from build123d import *

# Parameters (mm, degrees)
F0_R     = 1.5875
F1_DEPTH = 4.7625
F3_DEPTH = 58.1406
F5_DEPTH = 69.215
F7_DEPTH = 25.4
F9_DEPTH = 4.7625


with BuildPart() as f1:
    # F0 (on Top) → F1 (new body)
    with BuildSketch(Plane.XY):
        Polygon((-17.145, 87.89836), (-42.545, 87.89836), (-42.545, 0), (-45.72, 0), (-45.72, -58.15164), (-42.545, -58.15164), (-42.545, -66.08914), (-34.6075, -66.08914), (-34.6075, -69.26414), (34.6075, -69.26414), (34.6075, -66.08914), (42.545, -66.08914), (42.545, -58.15164), (45.72, -58.15164), (45.72, 0), (42.545, 0), (42.545, 87.89836), (17.145, 87.89836), (17.145, 27.487862), (12.7, 27.487862), (12.7, 91.07336), (-12.7, 91.07336), (-12.7, 27.487862), (-17.145, 27.487862), align=None)
        with Locations((-31.75, -43.86414)):
            Circle(F0_R, mode=Mode.SUBTRACT)
        with Locations((31.75, -43.86414)):
            Circle(F0_R, mode=Mode.SUBTRACT)
        with Locations((-31.75, 57.73586)):
            Circle(F0_R, mode=Mode.SUBTRACT)
        with Locations((31.75, 57.73586)):
            Circle(F0_R, mode=Mode.SUBTRACT)
    extrude(amount=F1_DEPTH)

    # F2 (on face) → F3 (join)
    with BuildSketch(Plane.XZ.offset(58.15164)):
        with BuildLine():
            Line((-45.72, 20.0025), (-45.72, 4.7625))
            Line((-45.72, 4.7625), (-42.545, 4.7625))
            Line((-42.545, 4.7625), (-42.545, 20.0025))
            ThreePointArc((-42.545, 20.0025), (-42.225108, 20.927946), (-41.402, 21.458299))
            ThreePointArc((-41.402, 21.458299), (-40.126284, 23.045799), (-41.402, 24.633299))
            ThreePointArc((-41.402, 24.633299), (-44.485221, 23.179692), (-45.72, 20.0025))
        make_face()
        with BuildLine():
            Line((42.545, 20.0025), (42.545, 4.7625))
            Line((42.545, 4.7625), (45.72, 4.7625))
            Line((45.72, 4.7625), (45.72, 20.0025))
            ThreePointArc((45.72, 20.0025), (44.485221, 23.179692), (41.402, 24.633299))
            ThreePointArc((41.402, 24.633299), (40.126284, 23.045799), (41.402, 21.458299))
            ThreePointArc((41.402, 21.458299), (42.225108, 20.927946), (42.545, 20.0025))
        make_face()
    extrude(amount=-F3_DEPTH)

    # F4 (on face) → F5 (join)
    with BuildSketch(Plane.YZ.offset(34.6075)):
        with BuildLine():
            Line((-69.26414, 20.0025), (-69.26414, 4.7625))
            Line((-69.26414, 4.7625), (-66.08914, 4.7625))
            Line((-66.08914, 4.7625), (-66.08914, 20.0025))
            ThreePointArc((-66.08914, 20.0025), (-65.769247, 20.927946), (-64.94614, 21.458299))
            ThreePointArc((-64.94614, 21.458299), (-63.670424, 23.045799), (-64.94614, 24.633299))
            ThreePointArc((-64.94614, 24.633299), (-68.029361, 23.179692), (-69.26414, 20.0025))
        make_face()
    extrude(amount=-F5_DEPTH)

    # F6 (on face) → F7 (join)
    with BuildSketch(Plane.YZ.offset(12.7)):
        with BuildLine():
            Line((87.89836, 4.7625), (91.07336, 4.7625))
            Line((91.07336, 4.7625), (91.07336, 9.5377))
            ThreePointArc((91.07336, 9.5377), (89.48586, 11.1252), (87.89836, 9.5377))
            Line((87.89836, 9.5377), (87.89836, 4.7625))
        make_face()
    extrude(amount=-F7_DEPTH)

    # F8 (on face) → F9 (cut)
    with BuildSketch(Plane.XY.offset(4.7625)):
        Polygon((-33.281147, 83.13586), (-37.7825, 83.13586), (-37.7825, 78.634507), align=None)
        Polygon((-21.9075, 81.039123), (-21.9075, 83.13586), (-26.545955, 83.13586), (-37.7825, 71.899315), (-37.7825, 65.164123), align=None)
        Polygon((-12.869341, 22.725362), (-19.604533, 22.725362), (-37.7825, 4.547394), (-37.7825, -2.187798), align=None)
        Polygon((34.070774, 83.13586), (27.335582, 83.13586), (21.9075, 77.707778), (21.9075, 70.972586), align=None)
        Polygon((37.7825, 73.377202), (37.7825, 80.112394), (21.9075, 64.237394), (21.9075, 57.502202), align=None)
        Polygon((31.047308, -61.32664), (37.7825, -61.32664), (37.7825, -54.591448), align=None)
        with BuildLine():
            Line((-37.7825, -49.334142), (-37.7825, -56.069335))
            Line((-37.7825, -56.069335), (37.7825, 19.495665))
            Line((37.7825, 19.495665), (37.7825, 26.230858))
            Line((37.7825, 26.230858), (-29.803871, -41.355513))
            ThreePointArc((-29.803871, -41.355513), (-29.504936, -46.109204), (-34.258626, -45.810269))
            Line((-34.258626, -45.810269), (-37.7825, -49.334142))
        make_face()
        with BuildLine():
            ThreePointArc((32.535156, 54.659474), (29.918155, 55.142606), (28.588111, 57.447621))
            Line((28.588111, 57.447621), (21.9075, 50.76701))
            Line((21.9075, 50.76701), (21.9075, 44.031818))
            Line((21.9075, 44.031818), (32.535156, 54.659474))
        make_face()
        with BuildLine():
            ThreePointArc((-33.990248, 55.485991), (-33.995064, 59.980924), (-29.50013, 59.976109))
            Line((-29.50013, 59.976109), (-21.9075, 67.568739))
            Line((-21.9075, 67.568739), (-21.9075, 74.303931))
            Line((-21.9075, 74.303931), (-37.7825, 58.428931))
            Line((-37.7825, 58.428931), (-37.7825, 51.693739))
            Line((-37.7825, 51.693739), (-33.990248, 55.485991))
        make_face()
        with BuildLine():
            Line((17.576924, -61.32664), (24.312116, -61.32664))
            Line((24.312116, -61.32664), (37.7825, -47.856255))
            Line((37.7825, -47.856255), (37.7825, -41.121063))
            Line((37.7825, -41.121063), (34.92286, -43.980704))
            ThreePointArc((34.92286, -43.980704), (33.995064, -46.109204), (31.866564, -47.036999))
            Line((31.866564, -47.036999), (17.576924, -61.32664))
        make_face()
        with BuildLine():
            Line((4.10654, -61.32664), (10.841732, -61.32664))
            Line((10.841732, -61.32664), (28.587678, -43.580694))
            ThreePointArc((28.587678, -43.580694), (29.504936, -41.619076), (31.466554, -40.701817))
            Line((31.466554, -40.701817), (37.7825, -34.385871))
            Line((37.7825, -34.385871), (37.7825, -27.650679))
            Line((37.7825, -27.650679), (4.10654, -61.32664))
        make_face()
        Polygon((-9.363845, -61.32664), (-2.628653, -61.32664), (37.7825, -20.915487), (37.7825, -14.180295), align=None)
        Polygon((-22.834229, -61.32664), (-16.099037, -61.32664), (37.7825, -7.445103), (37.7825, -0.709911), align=None)
        Polygon((-36.304613, -61.32664), (-29.569421, -61.32664), (37.7825, 6.025281), (37.7825, 12.760473), align=None)
        Polygon((-37.7825, -35.863758), (-37.7825, -42.59895), (37.7825, 32.96605), (37.7825, 39.701242), (20.80662, 22.725362), align=None)
        Polygon((-37.7825, -22.393374), (-37.7825, -29.128566), (14.071428, 22.725362), (7.336236, 22.725362), align=None)
        Polygon((-37.7825, -8.92299), (-37.7825, -15.658182), (0.601044, 22.725362), (-6.134148, 22.725362), align=None)
        Polygon((-37.7825, 18.017778), (-37.7825, 11.282586), (-21.9075, 27.157586), (-21.9075, 33.892778), align=None)
        Polygon((-37.7825, 31.488163), (-37.7825, 24.752971), (-21.9075, 40.627971), (-21.9075, 47.363163), align=None)
        Polygon((-37.7825, 44.958547), (-37.7825, 38.223355), (-21.9075, 54.098355), (-21.9075, 60.833547), align=None)
        Polygon((37.7825, 46.436434), (37.7825, 53.171626), (21.9075, 37.296626), (21.9075, 30.561434), align=None)
        with BuildLine():
            Line((37.7825, 59.906818), (37.7825, 66.64201))
            Line((37.7825, 66.64201), (32.038239, 60.89775))
            ThreePointArc((32.038239, 60.89775), (34.343254, 59.567706), (34.826387, 56.950705))
            Line((34.826387, 56.950705), (37.7825, 59.906818))
        make_face()
    extrude(amount=-F9_DEPTH, mode=Mode.SUBTRACT)


solid = f1.part
The model under review builds one solid part; all positions refer to its coordinate system, in mm. A direction names the side the tool comes from. Give positions to 0.01 mm unless a question says otherwise; leave off trailing zeros. Loops run counter-clockwise (first coordinate to the right, second up) from the corner with the lowest first, then second, coordinate; pieces in that order, holes last. Notation, with made-up numbers: (-20.5, -24) -> (8.5, -24) arc R12 ccw to (8.5, -9) -> close; hole circle Ø3 at (-15, 37.25). An arc over 180 degrees is marked (long way). Answer as a JSON object with one key per item and string values. Group by question number.
Q1. Draft analysis for pull direction X (two halves, no side actions). For faces 4 (the flat face through (-12.7, 59, 3)), 5 (the flat face through (-39, -66.089, 2)), state which applies: pulls with the +X half, pulls with the -X half, needs draft (parallel to the pull), parting line crosses it, or undercut.
Q2. Take a section at D-D (y = 62.5). Write out the cut boundary in (x, z) (1 decimal).
Q3. Take a section at B-B (z = 6.75). Write out the cut boundary in (x, y) (1 decimal), plus the area to 3 significant figures.
Q4. Take a section at A-A (z = 17.5). Write out the cut boundary in (x, y) (1 decimal), plus the area to 3 significant figures.
Q5. Take a section at C-C (y = 2.5). Write out the cut boundary in (x, z) (1 decimal), plus the area to 3 significant figures.
Q6. Insertion check: pin 1 (1.4 mm diameter, centred on y = 9, z = 1.5, fed in from -X) (3 decimals); pin 2 (1 mm diameter, centred on x = 25.5, y = 66, fed in from +Z); pin 3 (12 mm diameter, centred on y = 45, z = 4.5, fed in from +X) (3 decimals). Each pin has a flat end and moves straight along its axis. Give the tip position at first contact, or say it passes through.
Q7. Tool access review of faces 1 (the flat face through (-29.956, 19.109, 2.415)), 2 (the flat face through (17.145, 58, 2)), 3 (the flat face through (-44, -0.011, 15)): name each direction out of +Z, -Z, +X, -X, +Y, -Y from which nothing blocks a thin tool from reaching the whole face with its end or side.
Q8. Wall thickness on line 1 along X through (y, z) = (-10.5, 16.75) (3 decimals); line 2 along Y through (x, z) = (17.5, 17.5); line 3 along X through (y, z) = (76, 1.75) (1 decimal): over which ranges is each line inside the solid? List them lowest first.
Answer below:
{
 "1": {"face 4": "undercut", "face 5": "needs draft"},
 "2": {"outline": "(-42.5, 0) -> (-33.7, 0) -> (-33.7, 4.8) -> (-42.5, 4.8) -> close; (-27, 0) -> (-17.1, 0) -> (-17.1, 4.8) -> (-27, 4.8) -> close; (-12.7, 0) -> (12.7, 0) -> (12.7, 4.8) -> (-12.7, 4.8) -> close; (17.1, 0) -> (21.9, 0) -> (21.9, 4.8) -> (17.1, 4.8) -> close; (26.9, 0) -> (33.6, 0) -> (33.6, 4.8) -> (26.9, 4.8) -> close; (37.8, 0) -> (42.5, 0) -> (42.5, 4.8) -> (37.8, 4.8) -> close"},
 "3": {"outline": "(-45.7, -58.2) -> (-42.5, -58.2) -> (-42.5, 0) -> (-45.7, 0) -> close; (-34.6, -69.3) -> (34.6, -69.3) -> (34.6, -66.1) -> (-34.6, -66.1) -> close; (-12.7, 87.9) -> (12.7, 87.9) -> (12.7, 91.1) -> (-12.7, 91.1) -> close; (42.5, -58.2) -> (45.7, -58.2) -> (45.7, 0) -> (42.5, 0) -> close", "area": "670 mm2"},
 "4": {"outline": "(-45.7, -58.2) -> (-42.5, -58.2) -> (-42.5, 0) -> (-45.7, 0) -> close; (-34.6, -69.3) -> (34.6, -69.3) -> (34.6, -66.1) -> (-34.6, -66.1) -> close; (42.5, -58.2) -> (45.7, -58.2) -> (45.7, 0) -> (42.5, 0) -> close", "area": "589 mm2"},
 "5": {"outline": "(-42.5, 0) -> (-37.8, 0) -> (-37.8, 4.8) -> (-42.5, 4.8) -> close; (-33.1, 0) -> (-26.4, 0) -> (-26.4, 4.8) -> (-33.1, 4.8) -> close; (-19.6, 0) -> (-12.9, 0) -> (-12.9, 4.8) -> (-19.6, 4.8) -> close; (-6.2, 0) -> (0.6, 0) -> (0.6, 4.8) -> (-6.2, 4.8) -> close; (7.3, 0) -> (14.1, 0) -> (14.1, 4.8) -> (7.3, 4.8) -> close; (20.8, 0) -> (27.5, 0) -> (27.5, 4.8) -> (20.8, 4.8) -> close; (34.3, 0) -> (42.5, 0) -> (42.5, 4.8) -> (34.3, 4.8) -> close", "area": "223 mm2"},
 "6": {"pin 1": "stops at x = -42.545", "pin 2": "passes through", "pin 3": "stops at x = 42.545"},
 "7": {"face 1": "+Z, -Z", "face 2": "+Z, -Z, +Y", "face 3": "+Z, +X, -X, +Y"},
 "8": {"line 1": "x = -45.72 to -42.545, 42.545 to 45.72", "line 2": "y = -69.26 to -66.09", "line 3": "x = -42.5 to -33.7, -26.9 to -17.1, -12.7 to 12.7, 17.1 to 21.9, 26.9 to 33.7, 37.8 to 42.5"}
}
